from build123d import *

# Parameters (mm, degrees)
BOSS_EXTRUDE1_DEPTH      = 17.78
CUT_EXTRUDE1_DEPTH       = 12.7
BOSS_EXTRUDE2_DEPTH      = 5.08
BOSS_EXTRUDE2_DEPTH_BACK = 17.78
CUT_EXTRUDE2_REACH       = 93.511
SKETCH8_W                = 23.622
SKETCH8_H                = 33.02
CUT_EXTRUDE3_REACH       = 116.975
SKETCH9_W                = 7.62
SKETCH9_H                = 12.192
SKETCH10_W               = 15.24
SKETCH10_H               = 12.7
CUT_EXTRUDE4_DEPTH       = 5.08
SKETCH11_R               = 11.43
BOSS_EXTRUDE3_DEPTH      = 2.54


with BuildPart() as part:
    # Sketch1 → Boss-Extrude1 (new body)
    with BuildSketch(Plane.XY.offset(2.54)):
        with BuildLine():
            Line((-35.052, 0), (35.052, 0))
            ThreePointArc((35.052, 0), (37.207261469, 0.892738531), (38.1, 3.048))
            Line((38.1, 3.048), (38.1, 10.922))
            ThreePointArc((38.1, 10.922), (37.207261469, 13.077261469), (35.052, 13.97))
            Line((35.052, 13.97), (31.242, 13.97))
            ThreePointArc((31.242, 13.97), (29.086738531, 14.862738531), (28.194, 17.018))
            Line((28.194, 17.018), (28.194, 45.974))
            ThreePointArc((28.194, 45.974), (29.086738531, 48.129261469), (31.242, 49.022))
            Line((31.242, 49.022), (35.052, 49.022))
            ThreePointArc((35.052, 49.022), (37.207261469, 49.914738531), (38.1, 52.07))
            Line((38.1, 52.07), (38.1, 56.642))
            ThreePointArc((38.1, 56.642), (32.371594426, 70.471594426), (18.542, 76.2))
            Line((18.542, 76.2), (-18.542, 76.2))
            ThreePointArc((-18.542, 76.2), (-32.371594426, 70.471594426), (-38.1, 56.642))
            Line((-38.1, 56.642), (-38.1, 52.07))
            ThreePointArc((-38.1, 52.07), (-37.207261469, 49.914738531), (-35.052, 49.022))
            Line((-35.052, 49.022), (-31.242, 49.022))
            ThreePointArc((-31.242, 49.022), (-29.086738531, 48.129261469), (-28.194, 45.974))
            Line((-28.194, 45.974), (-28.194, 17.018))
            ThreePointArc((-28.194, 17.018), (-29.086738531, 14.862738531), (-31.242, 13.97))
            Line((-31.242, 13.97), (-35.052, 13.97))
            ThreePointArc((-35.052, 13.97), (-37.207261469, 13.077261469), (-38.1, 10.922))
            Line((-38.1, 10.922), (-38.1, 3.048))
            ThreePointArc((-38.1, 3.048), (-37.207261469, 0.892738531), (-35.052, 0))
        make_face()
    extrude(amount=-BOSS_EXTRUDE1_DEPTH)

    # Sketch2 → Cut-Extrude1 (cut)
    with BuildSketch(Plane(origin=(0, 0, -15.24), x_dir=(-1, 0, 0), z_dir=(0, 0, -1))):
        with BuildLine():
            Line((33.02, 54.102), (33.02, 56.642))
            ThreePointArc((33.02, 56.642), (28.779491978, 66.879491978), (18.542, 71.12))
            Line((18.542, 71.12), (-18.542, 71.12))
            ThreePointArc((-18.542, 71.12), (-28.779491978, 66.879491978), (-33.02, 56.642))
            Line((-33.02, 56.642), (-33.02, 54.102))
            Line((-33.02, 54.102), (-31.242, 54.102))
            ThreePointArc((-31.242, 54.102), (-25.494636083, 51.721363917), (-23.114, 45.974))
            Line((-23.114, 45.974), (-23.114, 17.018))
            ThreePointArc((-23.114, 17.018), (-25.494636083, 11.270636083), (-31.242, 8.89))
            Line((-31.242, 8.89), (-33.02, 8.89))
            Line((-33.02, 8.89), (-33.02, 5.08))
            Line((-33.02, 5.08), (33.02, 5.08))
            Line((33.02, 5.08), (33.02, 8.89))
            Line((33.02, 8.89), (31.242, 8.89))
            ThreePointArc((31.242, 8.89), (25.494636083, 11.270636083), (23.114, 17.018))
            Line((23.114, 17.018), (23.114, 45.974))
            ThreePointArc((23.114, 45.974), (25.494636083, 51.721363917), (31.242, 54.102))
            Line((31.242, 54.102), (33.02, 54.102))
        make_face()
    extrude(amount=-CUT_EXTRUDE1_DEPTH, mode=Mode.SUBTRACT)

    # Sketch7 → Boss-Extrude2 (add, two sides: drawn at the far end of the back side and taken through both)
    with BuildSketch(Plane(origin=(0, 0, -15.24), x_dir=(-1, 0, 0), z_dir=(0, 0, -1)).offset(-BOSS_EXTRUDE2_DEPTH_BACK)):
        with BuildLine():
            Line((18.542, 78.74), (-18.542, 78.74))
            ThreePointArc((-18.542, 78.74), (-34.167645651, 72.267645651), (-40.64, 56.642))
            Line((-40.64, 56.642), (-40.64, 52.07))
            ThreePointArc((-40.64, 52.07), (-39.003312693, 48.118687307), (-35.052, 46.482))
            Line((-35.052, 46.482), (-31.242, 46.482))
            ThreePointArc((-31.242, 46.482), (-30.882789755, 46.333210245), (-30.734, 45.974))
            Line((-30.734, 45.974), (-30.734, 17.018))
            ThreePointArc((-30.734, 17.018), (-30.882789755, 16.658789755), (-31.242, 16.51))
            Line((-31.242, 16.51), (-35.052, 16.51))
            ThreePointArc((-35.052, 16.51), (-39.003312693, 14.873312693), (-40.64, 10.922))
            Line((-40.64, 10.922), (-40.64, 3.048))
            ThreePointArc((-40.64, 3.048), (-39.003312693, -0.903312693), (-35.052, -2.54))
            Line((-35.052, -2.54), (35.052, -2.54))
            ThreePointArc((35.052, -2.54), (39.003312693, -0.903312693), (40.64, 3.048))
            Line((40.64, 3.048), (40.64, 10.922))
            ThreePointArc((40.64, 10.922), (39.003312693, 14.873312693), (35.052, 16.51))
            Line((35.052, 16.51), (31.242, 16.51))
            ThreePointArc((31.242, 16.51), (30.882789755, 16.658789755), (30.734, 17.018))
            Line((30.734, 17.018), (30.734, 45.974))
            ThreePointArc((30.734, 45.974), (30.882789755, 46.333210245), (31.242, 46.482))
            Line((31.242, 46.482), (35.052, 46.482))
            ThreePointArc((35.052, 46.482), (39.003312693, 48.118687307), (40.64, 52.07))
            Line((40.64, 52.07), (40.64, 56.642))
            ThreePointArc((40.64, 56.642), (34.167645651, 72.267645651), (18.542, 78.74))
        make_face()
        with BuildLine():
            ThreePointArc((-38.1, 52.07), (-37.207261469, 49.914738531), (-35.052, 49.022))
            Line((-35.052, 49.022), (-31.242, 49.022))
            ThreePointArc((-31.242, 49.022), (-29.086738531, 48.129261469), (-28.194, 45.974))
            Line((-28.194, 45.974), (-28.194, 17.018))
            ThreePointArc((-28.194, 17.018), (-29.086738531, 14.862738531), (-31.242, 13.97))
            Line((-31.242, 13.97), (-35.052, 13.97))
            ThreePointArc((-35.052, 13.97), (-37.207261469, 13.077261469), (-38.1, 10.922))
            Line((-38.1, 10.922), (-38.1, 3.048))
            ThreePointArc((-38.1, 3.048), (-37.207261469, 0.892738531), (-35.052, 0))
            Line((-35.052, 0), (35.052, 0))
            ThreePointArc((35.052, 0), (37.207261469, 0.892738531), (38.1, 3.048))
            Line((38.1, 3.048), (38.1, 10.922))
            ThreePointArc((38.1, 10.922), (37.207261469, 13.077261469), (35.052, 13.97))
            Line((35.052, 13.97), (31.242, 13.97))
            ThreePointArc((31.242, 13.97), (29.086738531, 14.862738531), (28.194, 17.018))
            Line((28.194, 17.018), (28.194, 45.974))
            ThreePointArc((28.194, 45.974), (29.086738531, 48.129261469), (31.242, 49.022))
            Line((31.242, 49.022), (35.052, 49.022))
            ThreePointArc((35.052, 49.022), (37.207261469, 49.914738531), (38.1, 52.07))
            Line((38.1, 52.07), (38.1, 56.642))
            ThreePointArc((38.1, 56.642), (32.371594426, 70.471594426), (18.542, 76.2))
            Line((18.542, 76.2), (-18.542, 76.2))
            ThreePointArc((-18.542, 76.2), (-32.371594426, 70.471594426), (-38.1, 56.642))
            Line((-38.1, 56.642), (-38.1, 52.07))
        make_face(mode=Mode.SUBTRACT)
    extrude(amount=BOSS_EXTRUDE2_DEPTH + BOSS_EXTRUDE2_DEPTH_BACK)

    # Cut-Extrude2: up to this face of the body (flat: up to its plane)
    cut_extrude2_end = Plane(part.part.faces().sort_by_distance((0, 37.604047464, 2.54))[0])
    # Sketch8 → Cut-Extrude2 (cut, up to the picked face)
    with BuildSketch(Plane(origin=(0, 0, -20.32), x_dir=(-1, 0, 0), z_dir=(0, 0, -1)), mode=Mode.PRIVATE) as cut_extrude2_sk1:
        with Locations((-34.671, 33.02)):
            Rectangle(SKETCH8_W, SKETCH8_H)
    cut_extrude2_tool1 = split(extrude(cut_extrude2_sk1.sketch, amount=-CUT_EXTRUDE2_REACH, mode=Mode.PRIVATE), bisect_by=cut_extrude2_end, keep=Keep.BOTH, mode=Mode.PRIVATE)
    # Sketch8 → Cut-Extrude2 (cut, up to the picked face)
    with BuildSketch(Plane(origin=(0, 0, -20.32), x_dir=(-1, 0, 0), z_dir=(0, 0, -1)), mode=Mode.PRIVATE) as cut_extrude2_sk2:
        with Locations((34.671, 33.02)):
            Rectangle(SKETCH8_W, SKETCH8_H)
    cut_extrude2_tool2 = split(extrude(cut_extrude2_sk2.sketch, amount=-CUT_EXTRUDE2_REACH, mode=Mode.PRIVATE), bisect_by=cut_extrude2_end, keep=Keep.BOTH, mode=Mode.PRIVATE)
    add(cut_extrude2_tool1.solids().sort_by(Axis((34.671, 33.02, -20.32), (0, 0, 1)))[0], mode=Mode.SUBTRACT)
    add(cut_extrude2_tool2.solids().sort_by(Axis((-34.671, 33.02, -20.32), (0, 0, 1)))[0], mode=Mode.SUBTRACT)

    # Cut-Extrude3: up to this face of the body (flat: up to its plane)
    cut_extrude3_end = Plane(part.part.faces().sort_by_distance((40.64, 6.985, -8.89))[0])
    # Sketch9 → Cut-Extrude3 (cut, up to the picked face)
    with BuildSketch(Plane.ZY.offset(40.64), mode=Mode.PRIVATE) as cut_extrude3_sk1:
        with Locations((-8.89, 6.096)):
            Rectangle(SKETCH9_W, SKETCH9_H)
    cut_extrude3_tool1 = split(extrude(cut_extrude3_sk1.sketch, amount=-CUT_EXTRUDE3_REACH, mode=Mode.PRIVATE), bisect_by=cut_extrude3_end, keep=Keep.BOTH, mode=Mode.PRIVATE)
    add(cut_extrude3_tool1.solids().sort_by(Axis((-40.64, 6.096, -8.89), (1, 0, 0)))[0], mode=Mode.SUBTRACT)

    # Sketch10 → Cut-Extrude4 (cut)
    with BuildSketch(Plane.XY.offset(2.54)):
        with Locations((0, 33.528)):
            Rectangle(SKETCH10_W, SKETCH10_H)
    extrude(amount=-CUT_EXTRUDE4_DEPTH, mode=Mode.SUBTRACT)

    # Sketch11 → Boss-Extrude3 (add)
    with BuildSketch(Plane.XY.offset(2.54)):
        with Locations((0.024363157, 61.722)):
            Circle(SKETCH11_R)
    extrude(amount=BOSS_EXTRUDE3_DEPTH)


solid = part.part
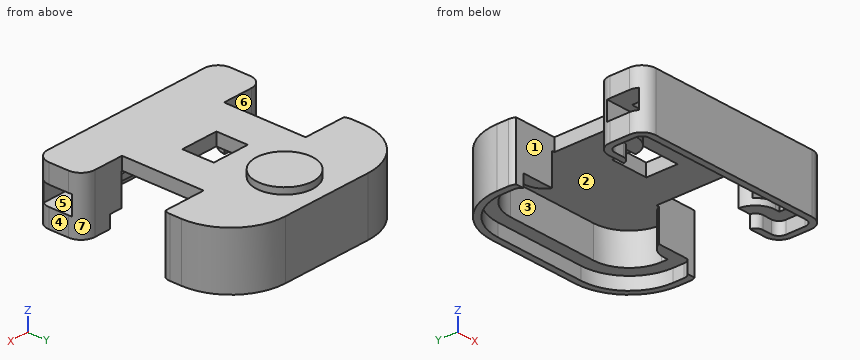
Input: part model. Units: mm. Frame: model coordinates. Face numbers are marked on the shaded views. A direction names the side the tool comes from. Coordinates: 2 decimals unless noted, no trailing zeros. Order: outer loops, then holes, each group sorted by start corner. A loop starts at its lowest first (then second) coordinate and runs counter-clockwise, first axis right, second up. Notation, with made-up numbers: M 24.25,-19.75 L 48.25,-19.75 A16 cw 48.25,4.25 Z; hole C 6,83 d10. An arc over 180 degrees is marked long. Answer in a Markdown table with one row per item.
(1) Section query B-B, the plane x = 4.5. Output: boundary loops of the cut face in (y, z), plus the area to 3 significant figures.
Numbers:
| item | result |
|---|---|
| outline | M -2.54,-20.32 L 0,-20.32 L 0,-15.24 L 5.08,-15.24 L 5.08,-12.7 L 0,-12.7 L 0,-5.08 L 5.08,-5.08 L 5.08,-2.54 L 27.18,-2.54 L 27.18,2.54 L -2.54,2.54 Z; M 39.88,-2.54 L 71.12,-2.54 L 71.12,-15.24 L 76.2,-15.24 L 76.2,-20.32 L 78.74,-20.32 L 78.74,2.54 L 72.24,2.54 L 72.24,5.08 L 51.2,5.08 L 51.2,2.54 L 39.88,2.54 Z |
| area | 582 mm^2 |
(2) Section query A-A, the plane z = -11. Give the number of separate pieces and of enclosed holes in the cut face, plus the area to 3 significant figures.
Numbers:
| item | result |
|---|---|
| separate pieces | 4 |
| enclosed holes | 0 |
| area | 1,220 mm^2 |
(3) Draft query along X for the marked faces 1, 2, 3 and 4. Return one class per face: pulls with the +X half, pulls with the -X half, needs draft (parallel to the pull), parting line crosses it, or undercut.
Numbers:
| item | result |
|---|---|
| face 1 | needs draft |
| face 2 | undercut |
| face 3 | undercut |
| face 4 | pulls with the +X half |
(4) Section query D-D, the plane x = -12.5. Output: boundary loops of the cut face in (y, z).
Numbers:
| item | result |
|---|---|
| outline | M -2.54,-20.32 L 0,-20.32 L 0,-15.24 L 5.08,-15.24 L 5.08,-12.7 L 0,-12.7 L 0,-5.08 L 5.08,-5.08 L 5.08,-2.54 L 71.12,-2.54 L 71.12,-15.24 L 76.2,-15.24 L 76.2,-20.32 L 78.74,-20.32 L 78.74,2.54 L -2.54,2.54 Z |
(5) Section query C-C, the plane y = 59. Output: boundary loops of the cut face in (x, z), plus the area to 3 significant figures.
Numbers:
| item | result |
|---|---|
| outline | M -40.51,-20.32 L -37.96,-20.32 L -37.96,-15.24 L -32.83,-15.24 L -32.83,-2.54 L 32.83,-2.54 L 32.83,-15.24 L 37.96,-15.24 L 37.96,-20.32 L 40.51,-20.32 L 40.51,2.54 L 11.13,2.54 L 11.13,5.08 L -11.08,5.08 L -11.08,2.54 L -40.51,2.54 Z |
| area | 689 mm^2 |
(6) Access query for the marked faces 5, 6 and 7. Directions: +Z, -Z, +X, -X, +Y, -Y. A direction counts if a zero-diameter tool reaches every point of the face in a straight line with its end or side. Return the directions, or none.
Numbers:
| item | result |
|---|---|
| face 5 | +X, -X |
| face 6 | +Z, -Z, -X |
| face 7 | +Z, -Z, +X |
(7) Contact query for flat-ended pins moving along their axis: pin 1 Ø2 at (x, y) = (-19, 27.5) entering from +Z; pin 2 Ø4 at (x, y) = (-9, 34) entering from -Z; pin 3 Ø0.9 at (x, z) = (32.5, -11.5) entering from +Y. Output: stop coordinate, or through.
Numbers:
| item | result |
|---|---|
| pin 1 | stops at z = 2.54 |
| pin 2 | stops at z = -2.54 |
| pin 3 | stops at y = 74.13 |
(8) Material intervals for line 1 (Z direction, x = 8, y = 4); line 2 (Y direction, x = -2, z = -18); line 3 (Y direction, x = 7.5, z = -12.25), sorted ascending. Write a range as [from, to].
Numbers:
| item | result |
|---|---|
| line 1 | z = [-15.24, -12.7], [-5.08, 2.54] |
| line 2 | y = [-2.54, 0], [76.2, 78.74] |
| line 3 | y = [-2.54, 0], [71.12, 78.74] |
